Input: part model. Units: mm. Frame: model coordinates. A direction names the side the tool comes from. Round coordinates to 2 decimals unless told otherwise and drop trailing zeros. Loops run counter-clockwise (first coordinate to the right, second up) from the corner with the lowest first, then second, coordinate; pieces in that order, holes last. Notation, with made-up numbers: (-20, 11.5) -> (-13, 11.5) arc R27 ccw to (-13, 48.5) -> close; hole circle Ø4 at (68, -21.5). An arc over 180 degrees is marked (long way). Answer as a JSON object with one key per item and string values. Group by question number.
Item 1: Section query D-D on z = 27. Return loops of the section in (x, y), and give its area (3 significant figures).
Item 2: Set-up query: faces 1 (the cylindrical face through (-85.12, -2.46, 60.74)), 2 (the cylindrical face through (-87.166, -2.465, -61.52)), 3 (the cylindrical face through (78.945, 1.479, 53.479)). Return all of +Z, -Z, +X, -X, +Y, -Y with unobstructed straight access to the full face (end or side cutting, diameter ignored); none if empty.
Item 3: Section query A-A on y = -2.5. Count the separate pieces of the cut face and the enclosed holes in it, and give its area (3 significant figures).
Item 4: Draft query along X for faces 4 (the cylindrical face through (86.52, -2.465, -62.166)), 5 (the cylindrical face through (-88.968, 1.479, 64.668)), 6 (the cylindrical face through (80.926, -21.199, -56.447)). Return one class per face: released by +X, released by -X, zero draft, split by the parting line, or undercut.
Item 5: Pin query (flat end, axial travel): pin 1 (1 mm diameter, centred on x = 47, z = 61.5, fed in from +Y); pin 2 (6 mm diameter, centred on x = -70, y = -6.5, fed in from +Z); pin 3 (10 mm diameter, centred on y = -38, z = 35, fed in from -X); pin 4 (2.5 mm diameter, centred on x = -6, y = -1.5, fed in from +Z). Return the tip coordinate at first contact, or that it passes through.
Item 6: Section query B-B on x = 8. Return loops of the section in (y, z), and give its area (3 significant figures).
Item 7: Material intervals for line 1 (X direction, y = -3, z = 32); line 2 (X direction, y = -30, z = 12.5); line 3 (Z direction, x = -32, y = -6), sorted ascending. Write a range as [from, to].
from build123d import *

# Parameters (mm, degrees)
BOSS_EXTRUDE1_DEPTH = 3
BOSS_EXTRUDE2_DEPTH = 5
BOSS_EXTRUDE3_DEPTH = 38
SKETCH4_W           = 22
SKETCH4_H           = 12
SKETCH4_W_2         = 20
SKETCH4_H_2         = 10
CUT_EXTRUDE1_DEPTH  = 461


with BuildPart() as part:
    # Sketch1 → Boss-Extrude1 (new body)
    with BuildSketch(Plane(origin=(0, 0, 0), x_dir=(1, 0, 0), z_dir=(0, 1, 0))):
        with BuildLine():
            ThreePointArc((-102.5, 32.5), (-89.319805153, 64.319805153), (-57.5, 77.5))
            Line((-57.5, 77.5), (57.5, 77.5))
            ThreePointArc((57.5, 77.5), (89.319805153, 64.319805153), (102.5, 32.5))
            Line((102.5, 32.5), (102.5, -32.5))
            ThreePointArc((102.5, -32.5), (89.319805153, -64.319805153), (57.5, -77.5))
            Line((57.5, -77.5), (-57.5, -77.5))
            ThreePointArc((-57.5, -77.5), (-89.319805153, -64.319805153), (-102.5, -32.5))
            Line((-102.5, -32.5), (-102.5, 32.5))
        make_face()
        with BuildLine():
            Line((-99, -32.5), (-99, 32.5))
            ThreePointArc((-99, 32.5), (-86.844931419, 61.844931419), (-57.5, 74))
            Line((-57.5, 74), (57.5, 74))
            ThreePointArc((57.5, 74), (86.844931419, 61.844931419), (99, 32.5))
            Line((99, 32.5), (99, -32.5))
            ThreePointArc((99, -32.5), (86.844931419, -61.844931419), (57.5, -74))
            Line((57.5, -74), (-57.5, -74))
            ThreePointArc((-57.5, -74), (-86.844931419, -61.844931419), (-99, -32.5))
        make_face(mode=Mode.SUBTRACT)
        with BuildLine():
            ThreePointArc((-99, 32.5), (-86.844931419, 61.844931419), (-57.5, 74))
            Line((-57.5, 74), (57.5, 74))
            ThreePointArc((57.5, 74), (86.844931419, 61.844931419), (99, 32.5))
            Line((99, 32.5), (99, -32.5))
            ThreePointArc((99, -32.5), (86.844931419, -61.844931419), (57.5, -74))
            Line((57.5, -74), (-57.5, -74))
            ThreePointArc((-57.5, -74), (-86.844931419, -61.844931419), (-99, -32.5))
            Line((-99, -32.5), (-99, 32.5))
        make_face()
        with BuildLine():
            Line((-97, -32.5), (-97, 32.5))
            ThreePointArc((-97, 32.5), (-85.430717857, 60.430717857), (-57.5, 72))
            Line((-57.5, 72), (57.5, 72))
            ThreePointArc((57.5, 72), (85.430717857, 60.430717857), (97, 32.5))
            Line((97, 32.5), (97, -32.5))
            ThreePointArc((97, -32.5), (85.430717857, -60.430717857), (57.5, -72))
            Line((57.5, -72), (-57.5, -72))
            ThreePointArc((-57.5, -72), (-85.430717857, -60.430717857), (-97, -32.5))
        make_face(mode=Mode.SUBTRACT)
        with BuildLine():
            ThreePointArc((-97, 32.5), (-85.430717857, 60.430717857), (-57.5, 72))
            Line((-57.5, 72), (57.5, 72))
            ThreePointArc((57.5, 72), (85.430717857, 60.430717857), (97, 32.5))
            Line((97, 32.5), (97, -32.5))
            ThreePointArc((97, -32.5), (85.430717857, -60.430717857), (57.5, -72))
            Line((57.5, -72), (-57.5, -72))
            ThreePointArc((-57.5, -72), (-85.430717857, -60.430717857), (-97, -32.5))
            Line((-97, -32.5), (-97, 32.5))
        make_face()
        with BuildLine():
            Line((-93, -32.5), (-93, 32.5))
            ThreePointArc((-93, 32.5), (-82.602290732, 57.602290732), (-57.5, 68))
            Line((-57.5, 68), (57.5, 68))
            ThreePointArc((57.5, 68), (82.602290732, 57.602290732), (93, 32.5))
            Line((93, 32.5), (93, -32.5))
            ThreePointArc((93, -32.5), (82.602290732, -57.602290732), (57.5, -68))
            Line((57.5, -68), (-57.5, -68))
            ThreePointArc((-57.5, -68), (-82.602290732, -57.602290732), (-93, -32.5))
        make_face(mode=Mode.SUBTRACT)
        with BuildLine():
            ThreePointArc((-93, 32.5), (-82.602290732, 57.602290732), (-57.5, 68))
            Line((-57.5, 68), (57.5, 68))
            ThreePointArc((57.5, 68), (82.602290732, 57.602290732), (93, 32.5))
            Line((93, 32.5), (93, -32.5))
            ThreePointArc((93, -32.5), (82.602290732, -57.602290732), (57.5, -68))
            Line((57.5, -68), (-57.5, -68))
            ThreePointArc((-57.5, -68), (-82.602290732, -57.602290732), (-93, -32.5))
            Line((-93, -32.5), (-93, 32.5))
        make_face()
        with BuildLine():
            Line((-87.5, -32.5), (-87.5, 32.5))
            ThreePointArc((-87.5, 32.5), (-78.713203436, 53.713203436), (-57.5, 62.5))
            Line((-57.5, 62.5), (57.5, 62.5))
            ThreePointArc((57.5, 62.5), (78.713203436, 53.713203436), (87.5, 32.5))
            Line((87.5, 32.5), (87.5, -32.5))
            ThreePointArc((87.5, -32.5), (78.713203436, -53.713203436), (57.5, -62.5))
            Line((57.5, -62.5), (-57.5, -62.5))
            ThreePointArc((-57.5, -62.5), (-78.713203436, -53.713203436), (-87.5, -32.5))
        make_face(mode=Mode.SUBTRACT)
        with BuildLine():
            ThreePointArc((-91, 32.5), (-81.18807717, 56.18807717), (-57.5, 66))
            Line((-57.5, 66), (57.5, 66))
            ThreePointArc((57.5, 66), (81.18807717, 56.18807717), (91, 32.5))
            Line((91, 32.5), (91, -32.5))
            ThreePointArc((91, -32.5), (81.18807717, -56.18807717), (57.5, -66))
            Line((57.5, -66), (-57.5, -66))
            ThreePointArc((-57.5, -66), (-81.18807717, -56.18807717), (-91, -32.5))
            Line((-91, -32.5), (-91, 32.5))
        make_face()
        with BuildLine():
            Line((-87.5, -32.5), (-87.5, 32.5))
            ThreePointArc((-87.5, 32.5), (-78.713203436, 53.713203436), (-57.5, 62.5))
            Line((-57.5, 62.5), (57.5, 62.5))
            ThreePointArc((57.5, 62.5), (78.713203436, 53.713203436), (87.5, 32.5))
            Line((87.5, 32.5), (87.5, -32.5))
            ThreePointArc((87.5, -32.5), (78.713203436, -53.713203436), (57.5, -62.5))
            Line((57.5, -62.5), (-57.5, -62.5))
            ThreePointArc((-57.5, -62.5), (-78.713203436, -53.713203436), (-87.5, -32.5))
        make_face(mode=Mode.SUBTRACT)
    extrude(amount=BOSS_EXTRUDE1_DEPTH)

    # Sketch1_4 → Boss-Extrude2 (add)
    with BuildSketch(Plane(origin=(0, 0, 0), x_dir=(1, 0, 0), z_dir=(0, 1, 0))):
        with BuildLine():
            ThreePointArc((-99, 32.5), (-86.844931419, 61.844931419), (-57.5, 74))
            Line((-57.5, 74), (57.5, 74))
            ThreePointArc((57.5, 74), (86.844931419, 61.844931419), (99, 32.5))
            Line((99, 32.5), (99, -32.5))
            ThreePointArc((99, -32.5), (86.844931419, -61.844931419), (57.5, -74))
            Line((57.5, -74), (-57.5, -74))
            ThreePointArc((-57.5, -74), (-86.844931419, -61.844931419), (-99, -32.5))
            Line((-99, -32.5), (-99, 32.5))
        make_face()
        with BuildLine():
            Line((-97, -32.5), (-97, 32.5))
            ThreePointArc((-97, 32.5), (-85.430717857, 60.430717857), (-57.5, 72))
            Line((-57.5, 72), (57.5, 72))
            ThreePointArc((57.5, 72), (85.430717857, 60.430717857), (97, 32.5))
            Line((97, 32.5), (97, -32.5))
            ThreePointArc((97, -32.5), (85.430717857, -60.430717857), (57.5, -72))
            Line((57.5, -72), (-57.5, -72))
            ThreePointArc((-57.5, -72), (-85.430717857, -60.430717857), (-97, -32.5))
        make_face(mode=Mode.SUBTRACT)
        with BuildLine():
            ThreePointArc((-93, 32.5), (-82.602290732, 57.602290732), (-57.5, 68))
            Line((-57.5, 68), (57.5, 68))
            ThreePointArc((57.5, 68), (82.602290732, 57.602290732), (93, 32.5))
            Line((93, 32.5), (93, -32.5))
            ThreePointArc((93, -32.5), (82.602290732, -57.602290732), (57.5, -68))
            Line((57.5, -68), (-57.5, -68))
            ThreePointArc((-57.5, -68), (-82.602290732, -57.602290732), (-93, -32.5))
            Line((-93, -32.5), (-93, 32.5))
        make_face()
        with BuildLine():
            Line((-91, -32.5), (-91, 32.5))
            ThreePointArc((-91, 32.5), (-81.18807717, 56.18807717), (-57.5, 66))
            Line((-57.5, 66), (57.5, 66))
            ThreePointArc((57.5, 66), (81.18807717, 56.18807717), (91, 32.5))
            Line((91, 32.5), (91, -32.5))
            ThreePointArc((91, -32.5), (81.18807717, -56.18807717), (57.5, -66))
            Line((57.5, -66), (-57.5, -66))
            ThreePointArc((-57.5, -66), (-81.18807717, -56.18807717), (-91, -32.5))
        make_face(mode=Mode.SUBTRACT)
    extrude(amount=-BOSS_EXTRUDE2_DEPTH)

    # Sketch2 → Boss-Extrude3 (add)
    with BuildSketch(Plane.XZ.offset(5)):
        with BuildLine():
            Line((-57.5, -68), (57.5, -68))
            ThreePointArc((57.5, -68), (82.602290732, -57.602290732), (93, -32.5))
            Line((93, -32.5), (93, 32.5))
            ThreePointArc((93, 32.5), (82.602290732, 57.602290732), (57.5, 68))
            Line((57.5, 68), (-57.5, 68))
            ThreePointArc((-57.5, 68), (-82.602290732, 57.602290732), (-93, 32.5))
            Line((-93, 32.5), (-93, -32.5))
            ThreePointArc((-93, -32.5), (-82.602290732, -57.602290732), (-57.5, -68))
        make_face()
        with BuildLine():
            Line((-91, 32.5), (-91, -32.5))
            ThreePointArc((-91, -32.5), (-81.18807717, -56.18807717), (-57.5, -66))
            Line((-57.5, -66), (57.5, -66))
            ThreePointArc((57.5, -66), (81.18807717, -56.18807717), (91, -32.5))
            Line((91, -32.5), (91, 32.5))
            ThreePointArc((91, 32.5), (81.18807717, 56.18807717), (57.5, 66))
            Line((57.5, 66), (-57.5, 66))
            ThreePointArc((-57.5, 66), (-81.18807717, 56.18807717), (-91, 32.5))
        make_face(mode=Mode.SUBTRACT)
    extrude(amount=BOSS_EXTRUDE3_DEPTH)

    # Sketch4 → Cut-Extrude1 (cut)
    with BuildSketch(Plane.XY.offset(68)):
        with Locations((-37.400499866, -25.448136165)):
            Rectangle(SKETCH4_W, SKETCH4_H)
        with Locations((-37.400499866, -25.448136165)):
            Rectangle(SKETCH4_W_2, SKETCH4_H_2, mode=Mode.SUBTRACT)
        with Locations((-37.400499866, -25.448136165)):
            Rectangle(SKETCH4_W_2, SKETCH4_H_2)
    extrude(amount=-CUT_EXTRUDE1_DEPTH, mode=Mode.SUBTRACT)


solid = part.part
Solved:
{
 "1": {"outline": "(-102.5, 0) -> (-99, 0) -> (-99, -5) -> (-97, -5) -> (-97, 0) -> (-93, 0) -> (-93, -43) -> (-91, -43) -> (-91, 0) -> (-87.5, 0) -> (-87.5, 3) -> (-102.5, 3) -> close; (87.5, 0) -> (91, 0) -> (91, -43) -> (93, -43) -> (93, 0) -> (97, 0) -> (97, -5) -> (99, -5) -> (99, 0) -> (102.5, 0) -> (102.5, 3) -> (87.5, 3) -> close", "area": "282 mm²"},
 "2": {"face 1": "-Y", "face 2": "-Z, -X, -Y", "face 3": "+Y, -Y"},
 "3": {"separate pieces": "2", "enclosed holes": "2", "area": "2,380 mm²"},
 "4": {"face 4": "released by +X", "face 5": "released by -X", "face 6": "undercut"},
 "5": {"pin 1": "through", "pin 2": "z = 72.8", "pin 3": "x = -93", "pin 4": "z = 74"},
 "6": {"outline": "(-43, -68) -> (0, -68) -> (0, -72) -> (-5, -72) -> (-5, -74) -> (0, -74) -> (0, -77.5) -> (3, -77.5) -> (3, -62.5) -> (0, -62.5) -> (0, -66) -> (-43, -66) -> close; (-43, 66) -> (0, 66) -> (0, 62.5) -> (3, 62.5) -> (3, 77.5) -> (0, 77.5) -> (0, 74) -> (-5, 74) -> (-5, 72) -> (0, 72) -> (0, 68) -> (-43, 68) -> close", "area": "282 mm²"},
 "7": {"line 1": "[-99, -97], [-93, -91], [91, 93], [97, 99]", "line 2": "[-93, -91], [91, 93]", "line 3": "[-68, -66], [66, 68]"}
}
